```python
from build123d import *

# Parameters (mm, degrees)
CROQUIS1_R                 = 5
SALIENTE_EXTRUIR1_DEPTH    = 339
CROQUIS8_R                 = 6.285812581
CORTAR_EXTRUIR5_DEPTH      = 163
CORTAR_EXTRUIR6_DEPTH      = 10
CORTAR_EXTRUIR6_DEPTH_BACK = 10
CROQUIS9_R                 = 2
CORTAR_EXTRUIR7_DEPTH      = 10
CORTAR_EXTRUIR7_DEPTH_BACK = 10
CROQUIS10_R                = 2


with BuildPart() as part:
    # Croquis1 → Saliente-Extruir1 (new body)
    with BuildSketch(Plane(origin=(0, 0, 0), x_dir=(1, 0, 0), z_dir=(0, 1, 0))):
        with Locations(Location((0, 0, 0), (0, 0, 270))):
            Circle(CROQUIS1_R)
    extrude(amount=SALIENTE_EXTRUIR1_DEPTH)

    # Croquis8 → Cortar-Extruir5 (cut)
    with BuildSketch(Plane.XZ):
        Circle(CROQUIS8_R)
    extrude(amount=-CORTAR_EXTRUIR5_DEPTH, mode=Mode.SUBTRACT)

    # Croquis9 → Cortar-Extruir6 (cut, two sides: drawn at the far end of the back side and taken through both)
    with BuildSketch(Plane.XY.offset(-CORTAR_EXTRUIR6_DEPTH_BACK)):
        with Locations(Location((0, 332.5, 0), (0, 0, 180))):
            Circle(CROQUIS9_R)
    extrude(amount=CORTAR_EXTRUIR6_DEPTH + CORTAR_EXTRUIR6_DEPTH_BACK, mode=Mode.SUBTRACT)

    # Croquis10 → Cortar-Extruir7 (cut, two sides: drawn at the far end of the back side and taken through both)
    with BuildSketch(Plane.XY.offset(-CORTAR_EXTRUIR7_DEPTH_BACK)):
        with Locations(Location((0, 169.5, 0), (0, 0, 180))):
            Circle(CROQUIS10_R)
    extrude(amount=CORTAR_EXTRUIR7_DEPTH + CORTAR_EXTRUIR7_DEPTH_BACK, mode=Mode.SUBTRACT)


solid = part.part
```
The listing builds one solid part. Answer for the finished solid, in the listing's coordinates (mm). Round coordinates to 2 decimals unless told otherwise and drop trailing zeros. Loops run counter-clockwise (first coordinate to the right, second up) from the corner with the lowest first, then second, coordinate; pieces in that order, holes last.
Q1. Find the intervals of material crossed by line 1 (Y direction, x = 0, z = 2.5); line 2 (X direction, y = 169.5, z = -0.5); line 3 (X direction, y = 332.5, z = 2.75), in increasing order.
Q2. Given pin 1 Ø1.5 at (y, z) = (255.5, 2.5) entering from -X; pin 2 Ø1 at (y, z) = (207, -3.5) entering from +X; pin 3 Ø3 at (y, z) = (321.5, -4) entering from +X, each flat-ended and moving along its own axis, determine where each tip first touches the part or whether it passes through.
Q3. For a pull along X with two mould halves and no side action, classify faces 1 (the face through (0, 339, 0)), 2 (the face through (-0.923, 171.274, -0.072)), 3 (the face through (-4.88, 249.77, -1.08)) as released by +X, released by -X, zero draft, split by the parting line, or undercut.
Q4. Section B-B, the plane y = 169.5 is taken. Determine the outline of the cut face in (x, z).
Q5. Section C-C, the plane y = 238.5 is taken. Determine the outline of the cut face in (x, z), then the cut area to 3 significant figures.
Q6. Section A-A, the plane x = 0 is taken. Determine the outline of the cut face in (y, z), then the cut area to 3 significant figures.
Completed:
1. line 1: y = 163 to 167.5, 171.5 to 330.5, 334.5 to 339
1. line 2: x = -4.97 to -2, 2 to 4.97
1. line 3: x = -4.18 to -2, 2 to 4.18
2. pin 1: stops at x = -4.68
2. pin 2: stops at x = 4
2. pin 3: stops at x = 4.33
3. face 1: zero draft
3. face 2: undercut
3. face 3: split by the parting line
4. outline: (-2, -4.58) - (-2, 4.58) arc R5 ccw to start; (2, -4.58) arc R5 ccw to (2, 4.58) - close
5. outline: circle Ø10 at (0, 0)
5. area: 78.5 mm2
6. outline: (163, -5) - (167.5, -5) - (167.5, 5) - (163, 5) - close; (171.5, -5) - (330.5, -5) - (330.5, 5) - (171.5, 5) - close; (334.5, -5) - (339, -5) - (339, 5) - (334.5, 5) - close
6. area: 1,680 mm2
